Could you check a few things on this model? Use its own coordinates, in mm. A direction names the side the tool comes from. Coordinates: 2 decimals unless noted, no trailing zeros. Write each loop counter-clockwise with the first axis right and the second up, starting at its lowest first coordinate (ties: lowest second). Pieces come first, ordered by that corner, then holes.
Item 1: If I drill on probe 1 along Y at (x, z) = (329, -100.5); probe 2 along Z at (x, y) = (-145, -1548); probe 3 along X at (y, z) = (-600, -171), over which ranges is the centre line in solid material (lowest first)?
Item 2: I want a section at C-C on x = 266.5. Please give me the cut outline in (y, z), then the cut area to 3 significant figures.
Item 3: Thinking about a two-plate mould opening in Z: for faces 3 (the cylindrical face through (291.9, -1605.5, -267.6)), 4 (the flat face through (-3, -1570, -3)), 5 (the cylindrical face through (-190.764, -809.5, -60.075)), 6 (the flat face through (6, -1640, -6)), which applies, +Z half, -Z half, draft (parallel to the pull), parting line (faces both ways), or undercut?
Item 4: I want a section at A-A on x = -41. Please give me the cut outline in (y, z).
Item 5: For P1, Ø1, axis at y = -397.5, z = 93.5, coming from the -X side; P2, Ø5, axis at y = -311.5, z = -113.5, coming from the -X side; P3, Ø4, axis at y = -1232.5, z = 41.5, coming from the +X side, each with a flat end and sliding along its axis, tell me the tip position at first contact or that it passes through.
Item 6: I want a section at B-B on y = -299. Please give me the cut outline in (x, z), then the cut area to 3 significant figures.
Item 7: Which directions (+Z, -Z, +X, -X, +Y, -Y) give clear straight access to the entire face, cutting with the end or side of a thin tool? Please do faces 1 (the cylindrical face through (249.76, -830.5, -10.99)), 2 (the flat face through (-6, 0, -6)).
from build123d import *

# Parameters (mm, degrees)
ESQUISSE2_R                  = 10
ENL_V_MAT_EXTRU_1_DEPTH      = 1733.983554452
R_P_TITION_CIRCULAIRE1_COUNT = 20


with BuildPart() as part:
    # Esquisse1 → Révolution1 (revolve)
    with BuildSketch(Plane.XY, mode=Mode.PRIVATE) as r_volution1_sk:
        Polygon((0, 0), (396, 0), (396, -70), (250, -70), (250, -1570), (396, -1570), (396, -1640), (0, -1640), (0, -1570), (200, -1570), (200, -70), (0, -70), align=None)
    revolve(r_volution1_sk.sketch.rotate(Axis((0, 0, 0), (0, -1, 0)), 180), axis=Axis((0, 0, 0), (0, -1, 0)))

    # Esquisse2 → Enlèv. mat.-Extru.1 (cut, through all)
    with BuildSketch(Plane(origin=(0, 0, 0), x_dir=(1, 0, 0), z_dir=(0, 1, 0))):
        with Locations(Location((366, 0, 0), (0, 0, 180))):
            Circle(ESQUISSE2_R)
    enl_v_mat_extru_1 = extrude(amount=-ENL_V_MAT_EXTRU_1_DEPTH, mode=Mode.SUBTRACT)

    # Répétition circulaire1: Enlèv. mat.-Extru.1 ×20 about axis
    r_p_tition_circulaire1_axis = Axis((0, 0, 0), (0, 1, 0))
    for i in range(1, R_P_TITION_CIRCULAIRE1_COUNT):
        add(enl_v_mat_extru_1.rotate(r_p_tition_circulaire1_axis, i * 360 / R_P_TITION_CIRCULAIRE1_COUNT), mode=Mode.SUBTRACT)


solid = part.part
Response values:
1. probe 1: y = -1640 to -1570, -70 to 0
1. probe 2: z = -203.65 to -137.75, 137.75 to 203.65
1. probe 3: x = -182.37 to -103.73, 103.73 to 182.37
2. outline: (-1640, -292.91) - (-1570, -292.91) - (-1570, 292.91) - (-1640, 292.91) - close; (-70, -292.91) - (0, -292.91) - (0, 292.91) - (-70, 292.91) - close
2. area: 82,000 mm2
3. face 3: parting line
3. face 4: undercut
3. face 5: undercut
3. face 6: draft
4. outline: (-1640, -393.87) - (-1570, -393.87) - (-1570, -246.62) - (-70, -246.62) - (-70, -393.87) - (0, -393.87) - (0, 393.87) - (-70, 393.87) - (-70, 246.62) - (-1570, 246.62) - (-1570, 393.87) - (-1640, 393.87) - close; hole (-1570, -195.75) - (-70, -195.75) - (-70, 195.75) - (-1570, 195.75) - close
5. P1: stops at x = -232.06
5. P2: stops at x = -224.01
5. P3: stops at x = 246.86
6. outline: circle Ø500 at (0, 0); hole circle Ø400 at (0, 0)
6. area: 70,700 mm2
7. face 1: none
7. face 2: +Z, -Z, +X, -X, +Y
